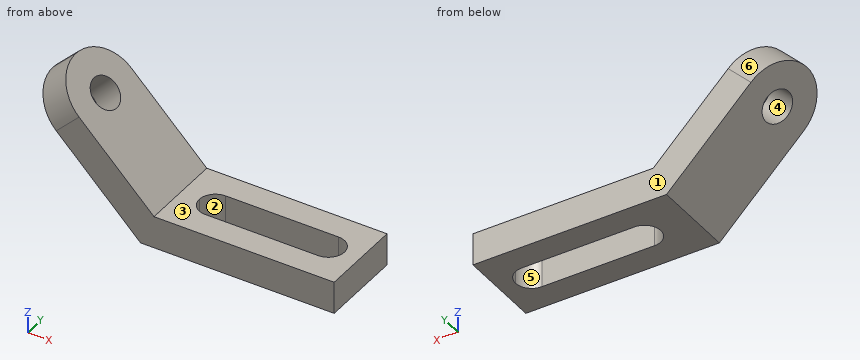
from build123d import *

# Parameters (mm, degrees)
F1_DEPTH = 52
F2_R     = 10
F3_DEPTH = 25
F4_R     = 25.99999
F6_DEPTH = 25
F7_R     = 9.99999


# Not quite as in the source:
# - a fillet or chamfer is up to 0.001 mm smaller than in the source, because OpenCascade refuses the exact size
# - a feature names something its author has since deleted; it is built from what else it names


with BuildPart() as f1:
    # F0 (on Front) → F1 (new body)
    with BuildSketch(Plane.XZ):
        Polygon((-120, 0), (0, 0), (0, 20), (-111.7157287525, 20), (-176.5685424949, 84.8528137424), (-190.7106781187, 70.7106781187), align=None)
    extrude(amount=F1_DEPTH)

    # F2 (on face) → F3 (cut)
    with BuildSketch(Plane(origin=(-45.8578643763, 0, -45.8578643763), x_dir=(0.7071067812, 0, -0.7071067812), z_dir=(0.7071067812, 0, 0.7071067812))):
        with Locations((-158.8528137424, -26)):
            Circle(F2_R)
    extrude(amount=-F3_DEPTH, mode=Mode.SUBTRACT)

    # F4 (radius 26 in the source; OpenCascade refuses exactly that, so slightly less here)
    f4_edges = [f1.edges().sort_by_distance(p)[0] for p in [
        (-183.63961, 0, 77.781746),
        (-183.63961, -52, 77.781746),
    ]]
    fillet(f4_edges, radius=F4_R)

    # F5 (on face) → F6 (cut)
    with BuildSketch(Plane.XY.offset(20)):
        Polygon((-10, -16), (-100, -16), (-100, -26), (-100, -36), (-10, -36), (-10, -26), align=None)
    extrude(amount=-F6_DEPTH, mode=Mode.SUBTRACT)

    # F7 (radius 10 in the source; OpenCascade refuses exactly that, so slightly less here)
    f7_edges = [f1.edges().sort_by_distance(p)[0] for p in [
        (-10, -16, 10),
        (-10, -36, 10),
        (-100, -16, 10),
        (-100, -36, 10),
    ]]
    fillet(f7_edges, radius=F7_R)


solid = f1.part
The listing builds one solid part. Answer for the finished solid, in the listing's coordinates (mm). Face numbers are marked on the shaded views. A direction names the side the tool comes from. Give positions to 0.01 mm unless a question says otherwise; leave off trailing zeros. Order: outer loops, then holes, each group sorted by start corner. A loop starts at its lowest first (then second) coordinate and runs counter-clockwise, first axis right, second up. Notation, with made-up numbers: (79, 78) -> (132, 78) arc R10 ccw to (132, 97) -> close; hole circle Ø8 at (-27.5, 40). An arc over 180 degrees is marked (long way). Put each result on its own line as item: value.
Item 1: Straight lines are drawn through the part: line 1 (Z direction, x = -54, y = -7); line 2 (X direction, y = -16, z = 24); line 3 (X direction, y = -12, z = 68.5). For each, find the intervals that lie inside material, in ascending order.
Established:
line 1: z = 0 to 20
line 2: x = -144 to -115.72
line 3: x = -187.14 to -160.22
Item 2: For the marked faces 1, 2 and 3, determine the directions among +Z, -Z, +X, -X, +Y, -Y from which every point of the face is accessible in a straight line to the end or side of a thin tool.
Established:
face 1: +Z, -Z, +X, -X, +Y
face 2: +Z, -Z
face 3: +Z, +X, +Y, -Y
Item 3: Given P1, Ø1, axis at x = -166.5, y = -36.5, coming from the -Z side; P2, Ø3, axis at x = -74, y = -9, coming from the +Z side; P3, Ø1.5, axis at x = -126, y = -20.5, coming from the -Z side, each flat-ended and moving along its own axis, determine where each tip first touches the part or whether it passes through.
Established:
P1: stops at z = 46
P2: stops at z = 20
P3: stops at z = 5.25
Item 4: A cutting plane is placed at A-A on x = -51. Give the vertices of the cut face in (y, z).
Established:
outline: (-52, 0) -> (-36, 0) -> (-36, 20) -> (-52, 20) -> close; (-16, 0) -> (0, 0) -> (0, 20) -> (-16, 20) -> close
Item 5: A cutting plane is placed at C-C on y = -20.5. Give the vertices of the cut face in (x, z), plus the area to 3 significant figures.
Established:
outline: (-190.29, 70.29) -> (-178.23, 58.23) -> (-164.09, 72.37) -> (-176.15, 84.44) -> close; (-166.42, 46.42) -> (-120, 0) -> (-98.35, 0) -> (-98.35, 20) -> (-111.72, 20) -> (-152.28, 60.56) -> close; (-11.65, 0) -> (0, 0) -> (0, 20) -> (-11.65, 20) -> close
area: 2,150 mm^2
Item 6: For a pull along Z with two mould halves and no side action, classify the marked faces 4, 5 and 6 as released by +Z, released by -Z, zero draft, split by the parting line, or undercut.
Established:
face 4: undercut
face 5: zero draft
face 6: released by +Z
Item 7: A cutting plane is placed at D-D on y = -44. Give the vertices of the cut face in (x, z).
Established:
outline: (-185.59, 65.59) -> (-120, 0) -> (0, 0) -> (0, 20) -> (-111.72, 20) -> (-171.45, 79.73) -> close
